from build123d import *

# Parameters (mm, degrees)
SKETCH_1_W      = 42
SKETCH_1_H      = 40
SKETCH_1_W_2    = 38
SKETCH_1_H_2    = 36
EXTRUDE_1_DEPTH = 27
FILLET_1_R      = 2.5


with BuildPart() as part:
    # 草图1 → 凸台-拉伸1 (new body)
    with BuildSketch(Plane(origin=(0, 0, 0), x_dir=(0, 0, -1), z_dir=(1, 0, 0))):
        Rectangle(SKETCH_1_W, SKETCH_1_H)
        Rectangle(SKETCH_1_W_2, SKETCH_1_H_2, mode=Mode.SUBTRACT)
    extrude(amount=EXTRUDE_1_DEPTH)

    # 圆角1
    fillet_1_edges = [part.edges().sort_by_distance(p)[0] for p in [
        (13.5, -18, -19),
        (13.5, 18, -19),
        (13.5, 18, 19),
        (13.5, -18, 19),
        (13.5, 20, 21),
        (13.5, 20, -21),
        (13.5, -20, -21),
        (13.5, -20, 21),
    ]]
    fillet(fillet_1_edges, radius=FILLET_1_R)


solid = part.part
Input: part model. Units: mm. Frame: model coordinates. A direction names the side the tool comes from. Give positions to 0.01 mm unless a question says otherwise; leave off trailing zeros. Order: outer loops, then holes, each group sorted by start corner. A loop starts at its lowest first (then second) coordinate and runs counter-clockwise, first axis right, second up.
Q1. Set-up query: faces 1 (the cylindrical face through (13.689, 17.248, -18.287)), 2 (the cylindrical face through (13.689, -19.287, -20.248)). Return all of +Z, -Z, +X, -X, +Y, -Y with unobstructed straight access to the full face (end or side cutting, diameter ignored); none if empty.
Checked values:
face 1: +X, -X
face 2: -Z, +X, -X, -Y
Q2. Ray query, probe 1 along Z at (x, y) = (15.5, 8); probe 2 along Y at (x, z) = (18, -8); probe 3 along Z at (x, y) = (4, 17). Return the intervals inside material, ascending.
Checked values:
probe 1: z = -21 to -19, 19 to 21
probe 2: y = -20 to -18, 18 to 20
probe 3: z = -21 to -18.5, 18.5 to 21
Q3. Section B-B on x = 18. Output: boundary loops of the cut face in (y, z), and give its area (3 significant figures).
Checked values:
outline: (-20, -18.5) arc R2.5 ccw to (-17.5, -21) - (17.5, -21) arc R2.5 ccw to (20, -18.5) - (20, 18.5) arc R2.5 ccw to (17.5, 21) - (-17.5, 21) arc R2.5 ccw to (-20, 18.5) - close; hole (-18, -16.5) arc R2.5 ccw to (-15.5, -19) - (15.5, -19) arc R2.5 ccw to (18, -16.5) - (18, 16.5) arc R2.5 ccw to (15.5, 19) - (-15.5, 19) arc R2.5 ccw to (-18, 16.5) - close
area: 312 mm2
Q4. Draft query along Y for faces 3 (the cylindrical face through (13.689, 17.287, 18.248)), 4 (the cylindrical face through (13.689, -19.248, 20.287)), 5 (the cylindrical face through (13.689, 19.248, 20.287)). Return one class per face: +Y half, -Y half, draft (parallel to the pull), parting line (faces both ways), or undercut.
Checked values:
face 3: undercut
face 4: -Y half
face 5: +Y half
Q5. Section C-C on z = 10. Output: boundary loops of the cut face in (x, y), and give its area (3 significant figures).
Checked values:
outline: (0, -20) - (27, -20) - (27, -18) - (0, -18) - close; (0, 18) - (27, 18) - (27, 20) - (0, 20) - close
area: 108 mm2
Q6. Section A-A on y = -11.5. Output: boundary loops of the cut face in (x, z), and give its area (3 significant figures).
Checked values:
outline: (0, -21) - (27, -21) - (27, -19) - (0, -19) - close; (0, 19) - (27, 19) - (27, 21) - (0, 21) - close
area: 108 mm2
